from build123d import *

# Parameters (mm, degrees)
F1_DEPTH = 19.05
F3_DEPTH = 9.525
F5_DEPTH = 9.525


# Not quite as in the source:
# - a feature names something its author has since deleted; it is built from what else it names


with BuildPart() as f1:
    # F0 (on Top) → F1 (new body)
    with BuildSketch(Plane.XY):
        with BuildLine():
            Line((727.2677384075, 427.9083177516), (727.2677384075, -283.5772421425))
            ThreePointArc((727.2677384075, -283.5772421425), (774.3773382982, -328.2348347436), (816.4554812019, -278.8076674308))
            Line((816.4554812019, -278.8076674308), (816.4554812019, -221.0955097314))
            Line((816.4554812019, -221.0955097314), (1159.4623036636, -98.9686407408))
            Line((1159.4623036636, -98.9686407408), (1178.6487772739, -128.0367093729))
            Line((1178.6487772739, -128.0367093729), (1189.3036458742, -145.3996676047))
            ThreePointArc((1189.3036458742, -145.3996676047), (1254.3589120262, -165.180351508), (1280.8355912672, -102.5508970465))
            Line((1280.8355912672, -102.5508970465), (881.2480453078, 396.8848219998))
            ThreePointArc((881.2480453078, 396.8848219998), (878.9075846932, 401.4943033077), (878.5980767553, 406.6546597539))
            Line((878.5980767553, 406.6546597539), (902.2401524871, 568.497452094))
            ThreePointArc((902.2401524871, 568.497452094), (903.8120375637, 573.0182606597), (906.9455405898, 576.6362285378))
            Line((906.9455405898, 576.6362285378), (941.9003890149, 604.1852707886))
            Line((941.9003890149, 604.1852707886), (899.3018677789, 723.8279303566))
            Line((899.3018677789, 723.8279303566), (891.7270738587, 721.1309406639))
            Line((891.7270738587, 721.1309406639), (888.532184766, 730.1041401315))
            Line((888.532184766, 730.1041401315), (557.8398737201, 612.361827435))
            Line((557.8398737201, 612.361827435), (561.0347628128, 603.3886279674))
            Line((561.0347628128, 603.3886279674), (540.3738890749, 596.0323666485))
            Line((540.3738890749, 596.0323666485), (584.2529836062, 476.853404314))
            Line((584.2529836062, 476.853404314), (710.1798289544, 523.2169221936))
            ThreePointArc((710.1798289544, 523.2169221936), (721.8328450807, 521.7157540947), (727.2677384075, 511.2990259602))
            Line((727.2677384075, 511.2990259602), (727.2677384075, 427.9083177516))
        make_face()
        with BuildLine():
            Line((1099.3852571882, -15.0422832395), (825.3589785984, -112.6087723988))
            Line((825.3589785984, -112.6087723988), (812.2279623998, 291.9047427935))
            ThreePointArc((812.2279623998, 291.9047427935), (820.3847868922, 304.1789193457), (834.6503380579, 300.4798321914))
            Line((834.6503380579, 300.4798321914), (1099.3852571882, -15.0422832395))
        make_face(mode=Mode.SUBTRACT)
    extrude(amount=F1_DEPTH)

    # F2 (on face) → F3 (cut)
    with BuildSketch(Plane.XY.offset(19.05)):
        with BuildLine():
            ThreePointArc((837.5686180204, -153.7290348884), (831.0198662622, -167.5195352567), (844.8103666306, -174.068287015))
            Line((844.8103666306, -174.068287015), (1131.9527495937, -71.8318360485))
            ThreePointArc((1131.9527495937, -71.8318360485), (1138.501501352, -58.0413356801), (1124.7110009836, -51.4925839219))
            Line((1124.7110009836, -51.4925839219), (837.5686180204, -153.7290348884))
        make_face()
    extrude(amount=-F3_DEPTH, mode=Mode.SUBTRACT)

    # F4 (on face) → F5 (cut)
    with BuildSketch(Plane.XY.offset(19.05)):
        Polygon((580.3132639661, 522.4942656533), (587.5549912453, 502.1550059319), (931.5862417023, 624.6462138439), (924.4067217173, 644.8107569177), (920.2038128035, 643.3143248671), (892.0960137021, 722.2584502232), (888.9011246094, 731.2316496908), (868.5033081007, 724.1565396792), (899.8030168616, 636.2475531691), align=None)
    extrude(amount=-F5_DEPTH, mode=Mode.SUBTRACT)


solid = f1.part
Verification items for the finished model (mm, model axes). A direction names the side the tool comes from. Give positions to 0.01 mm unless a question says otherwise; leave off trailing zeros. Order: outer loops, then holes, each group sorted by start corner. A loop starts at its lowest first (then second) coordinate and runs counter-clockwise, first axis right, second up. Notation, with made-up numbers: M 26,75 L 66,75 A20 cw 66,92 Z; hole C 8,-4.5 d2. An arc over 180 degrees is marked long. Answer as a JSON object with one key per item and string values. Group by question number.
1) Depth check by flat-ended pin: pin 1 Ø1 at (y, z) = (84, 12.5) entering from +X; pin 2 Ø9.5 at (y, z) = (-236.5, 13) entering from +X; pin 3 Ø1 at (x, z) = (850.5, 6.5) entering from -Y. Enter the tip coordinate at first touch or a pass-through.
2) Access from +Z, -Z, +X, -X, +Y, -Y to the whole of each face (thin tool, end or side, straight path). Record for faces 1 (the face through (646.33, 499.71, 9.39)), 2 (the face through (965.16, 144.93, 9.39)), 3 (the face through (884.124, 680.285, 14.354)).
3) Mould release check, pull along Y, two halves, no side actions. Record for faces 4 (the face through (562.006, 537.277, 9.392)), 5 (the face through (938, 243, 0)), 6 (the face through (983.15, -101.895, 14.354)): released by +Y, released by -Y, zero draft, split by the parting line, or undercut.
4) Cross-section at B-B (x = 1013.5). Enter the section's corners in (y, z) (3 decimals), then the cut area to 3 significant figures.
5) Scan lines: line 1 along Y through (x, z) = (865, 10.5); line 2 along Y through (x, z) = (867.5, 14.25); line 3 along Y through (x, z) = (994.5, 16). Record each from-to range of solid material in increasing order. Write a range as [from, to].
6) Cross-section at A-A (z = 6). Enter the section's corners in (x, y).
7) Cross-section at D-D (x = 772.5). Enter the section's corners in (y, z) (3 decimals).
8) Cross-section at C-C (y = 54.5). Enter the section's corners in (x, z).
Result sheet:
{
 "1": {"pin 1": "stops at x = 1131.98", "pin 2": "stops at x = 816.46", "pin 3": "stops at y = -209.15"},
 "2": {"face 1": "+Z, -Z, -Y", "face 2": "+Z, -Z", "face 3": "+Z"},
 "3": {"face 4": "released by -Y", "face 5": "zero draft", "face 6": "undercut"},
 "4": {"outline": "M -150.938,0 L -45.622,0 L -45.622,19.05 L -91.089,19.05 L -91.089,9.525 L -114.007,9.525 L -114.007,19.05 L -150.938,19.05 Z; M 87.319,0 L 231.586,0 L 231.586,19.05 L 87.319,19.05 Z", "area": "4,540 mm2"},
 "5": {"line 1": "y = [-203.81, -166.88], [-143.96, -98.49], [264.31, 600.94], [623.86, 721.73]", "line 2": "y = [-202.92, -165.99], [-143.07, -97.6], [261.33, 601.83], [624.75, 722.62]", "line 3": "y = [-157.7, -120.77], [-97.85, -52.39], [109.96, 255.33]"},
 "6": {"outline": "M 540.37,596.03 L 584.25,476.85 L 710.18,523.22 A12.7 cw 727.27,511.3 L 727.27,-283.58 A44.72 ccw long 816.46,-278.81 L 816.46,-221.1 L 1159.46,-98.97 L 1178.65,-128.04 L 1189.3,-145.4 A50.81 ccw 1280.84,-102.55 L 881.25,396.88 A12.7 cw 878.6,406.65 L 902.24,568.5 A12.7 cw 906.95,576.64 L 941.9,604.19 L 899.3,723.83 L 891.73,721.13 L 888.53,730.1 L 557.84,612.36 L 561.03,603.39 Z; hole M 812.23,291.9 L 825.36,-112.61 L 1099.39,-15.04 L 834.65,300.48 A12.7 ccw Z"},
 "7": {"outline": "M -328.296,0 L 688.791,0 L 688.791,19.05 L 590.922,19.05 L 590.922,9.525 L 568.004,9.525 L 568.004,19.05 L -328.296,19.05 Z"},
 "8": {"outline": "M 727.27,0 L 819.93,0 L 819.93,19.05 L 727.27,19.05 Z; M 1041.04,0 L 1155.18,0 L 1155.18,19.05 L 1041.04,19.05 Z"}
}
